Part model, mm, in its own coordinate system. Round coordinates to 2 decimals unless told otherwise and drop trailing zeros. Write each loop counter-clockwise with the first axis right and the second up, starting at its lowest first coordinate (ties: lowest second). Pieces come first, ordered by that corner, then holes.
from build123d import *

# Parameters (mm, degrees)
CUT_EXTRUDE1_DEPTH       = 16.362291496
CUT_EXTRUDE1_DEPTH_BACK  = 5
SKETCH2_W                = 5.5
SKETCH2_H                = 2.8
M3_CLEARANCE_HOLE1_D     = 3.2
M3_CLEARANCE_HOLE1_DEPTH = 1.5
BOSS_EXTRUDE1_DEPTH      = 4.3


with BuildPart() as part:
    # Sketch1 → Revolve1 (revolve)
    with BuildSketch(Plane(origin=(0, 0, 0), x_dir=(0, 0, -1), z_dir=(1, 0, 0))):
        with BuildLine():
            Line((0, 0), (0, 6))
            ThreePointArc((0, 6), (5.830951895, 4.384919825), (10, 0))
            Line((10, 0), (0, 0))
        make_face()
    revolve(axis=Axis((0, 0, 0), (0, 1, 0)))

    # Sketch2 → Cut-Extrude1 (cut, two sides: drawn at the far end of the back side and taken through both)
    with BuildSketch(Plane(origin=(0, 0, 0), x_dir=(0, 0, -1), z_dir=(1, 0, 0)).offset(-CUT_EXTRUDE1_DEPTH_BACK)):
        with Locations((0, 2.9)):
            Rectangle(SKETCH2_W, SKETCH2_H)
    extrude(amount=CUT_EXTRUDE1_DEPTH + CUT_EXTRUDE1_DEPTH_BACK, mode=Mode.SUBTRACT)

    # M3 Clearance Hole1
    with Locations(Plane(origin=(0, 0, 0), x_dir=(-1, 0, 0), z_dir=(0, -1, 0))):
        with Locations((0, 0)):
            Hole(M3_CLEARANCE_HOLE1_D / 2, depth=M3_CLEARANCE_HOLE1_DEPTH)

    # Sketch11 → Boss-Extrude1 (add)
    with BuildSketch(Plane(origin=(0, 0, 0), x_dir=(1, 0, 0), z_dir=(0, 1, 0))):
        with BuildLine():
            Line((5.29913515, 2.75), (-1.703183294, 2.95))
            Line((-1.703183294, 2.95), (-3.406366588, 0))
            Line((-3.406366588, 0), (-1.703183294, -2.95))
            Line((-1.703183294, -2.95), (5.29913515, -2.75))
            ThreePointArc((5.29913515, -2.75), (-5.970203793, 0), (5.29913515, 2.75))
        make_face()
    extrude(amount=BOSS_EXTRUDE1_DEPTH)


solid = part.part
Q1. Saw through at C-C, the plane y = 0.6. Write the cut outline in (x, z), and give its area (3 significant figures).
Q2. Saw through at B-B, the plane x = 0. Write the cut outline in (y, z), and give its area (3 significant figures).
Q3. Two-plate mould, pull along Y, no slides. Class faces 1 (the flat face through (4, 1.5, 0)), 2 (the flat face through (-2, 0, 0)), 3 (the flat face through (-2.6, 2.9, 1.4)), 4 (the cylindrical face through (-1.27, 0.76, 0.97)): released by +Y, released by -Y, zero draft, split by the parting line, or undercut.
Q4. Wall check: line 1 (Z direction, x = 4.25, y = 1.8); line 2 (Z direction, x = 5, y = 1.75); line 3 (Y direction, x = 2, z = 2.25). Give the ranges that are in metal, low to high.
Q5. Saw through at D-D, the plane z = 2.5. Write the cut outline in (x, y), and give its area (3 significant figures).
Q6. Saw through at A-A, the plane x = -3. Write the cut outline in (y, z), and give its area (3 significant figures).
Q7. Drop flat-ended pins along their axis: P1, Ø1.9, axis at x = 0, z = 0, coming from the -Y side; P2, Ø2, axis at x = 4, y = 2.5, coming from the +Z side; P3, Ø1.5, axis at y = 4.5, z = 8, coming from the -X side; P4, Ø3, axis at y = 2, z = -0.5, coming from the -X side. Give the stop position or say it passes through.
Computed:
1. outline: circle Ø19.31 at (0, 0); hole circle Ø3.2 at (0, 0)
1. area: 285 mm2
2. outline: (0, -10) arc R11.33 ccw to (0, 10) - (0, 1.6) - (1.5, 1.6) - (1.5, 2.75) - (4.3, 2.75) - (4.3, -2.75) - (1.5, -2.75) - (1.5, -1.6) - (0, -1.6) - close
2. area: 65.3 mm2
3. face 1: undercut
3. face 2: released by -Y
3. face 3: undercut
3. face 4: zero draft
4. line 1: z = -7.71 to -2.75, 2.75 to 7.71
4. line 2: z = -7.3 to -2.75, 2.75 to 7.3
4. line 3: y = 0 to 1.5, 4.3 to 5.59
5. outline: (-9.68, 0) - (9.68, 0) arc R11.05 ccw to (8.69, 1.5) - (-1.96, 1.5) - (-1.96, 4.3) - (5.42, 4.3) arc R11.05 ccw to start
5. area: 52.9 mm2
6. outline: (0, -9.54) arc R10.93 ccw to (0, 9.54) - close; hole (1.5, -0.7) - (4.3, -0.7) - (4.3, 0.7) - (1.5, 0.7) - close
6. area: 71.9 mm2
7. P1: stops at y = 4.3
7. P2: stops at z = 8.23
7. P3: passes through
7. P4: stops at x = -9.71
